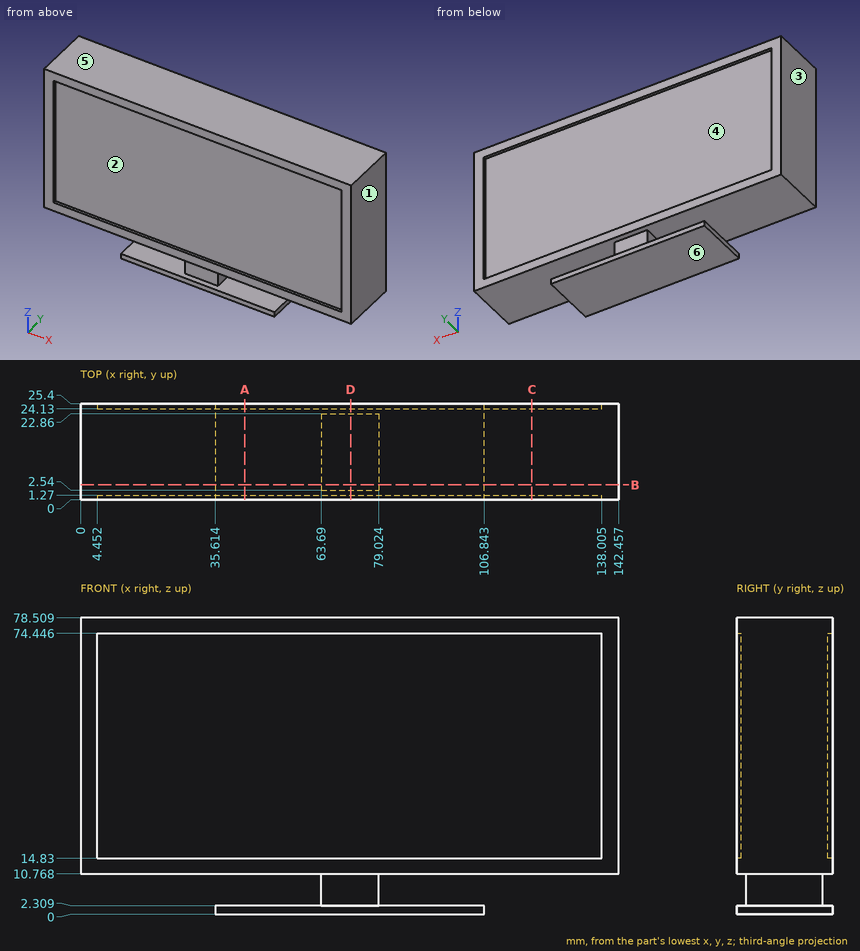
Verification items for this drawing (mm, ordinates from the low corner). A direction names the side the tool comes from. Round coordinates to 2 decimals unless told otherwise and drop trailing zeros. Order: outer loops, then holes, each group sorted by start corner. A loop starts at its lowest first (then second) coordinate and runs counter-clockwise, first axis right, second up. Notation, with made-up numbers: (23.25, 17.25) - (63.25, 17.25) arc R19 ccw to (63.25, 52.25) - close; hole circle Ø6 at (75, -34.5). An arc over 180 degrees is marked (long way). Use CSV: the item, a comma, the result in double quotes.
(1) Access from +Z, -Z, +X, -X, +Y, -Y to the whole of each face (thin tool, end or side, straight path). Record for the marked faces 1 and 2.
Entries:
face 1,"+Z, -Z, +X, +Y, -Y"
face 2,"-Y"
(2) Section check A-A on x = 43.5. Record the boundary of the cut face in (y, z) (1 decimal), and give its area (3 significant figures).
Entries:
outline,"(0, 0) - (25.4, 0) - (25.4, 2.3) - (0, 2.3) - close; (0, 10.8) - (25.4, 10.8) - (25.4, 14.8) - (24.1, 14.8) - (24.1, 74.4) - (25.4, 74.4) - (25.4, 78.5) - (0, 78.5) - (0, 74.4) - (1.3, 74.4) - (1.3, 14.8) - (0, 14.8) - close"
area,"1,630 mm^2"
(3) Gauge pin test, flat ends, axial feed: pin 1 Ø4 at (y, z) = (15.5, 6) entering from +X; pin 2 Ø4 at (x, z) = (70, 5) entering from -Y; pin 3 Ø2.5 at (y, z) = (8.5, 7.5) entering from -X. Record the tip position at first contact, or that the pin passes through.
Entries:
pin 1,"x = 79.02"
pin 2,"y = 2.54"
pin 3,"x = 63.69"
(4) Section check B-B on y = 4. Record the boundary of the cut face in (x, z) (1 decimal).
Entries:
outline,"(0, 10.8) - (63.7, 10.8) - (63.7, 2.3) - (35.6, 2.3) - (35.6, 0) - (106.8, 0) - (106.8, 2.3) - (79, 2.3) - (79, 10.8) - (142.5, 10.8) - (142.5, 78.5) - (0, 78.5) - close"
(5) Thickness scan on probe 1 along Z at (x, y) = (41, 13.5); probe 2 along Z at (x, y) = (11.5, 7.75); probe 3 along Y at (x, z) = (63.5, 30.5). Record the ranges inside material, lowest first. Write a range as from..to.
Entries:
probe 1,"0..2.31, 10.77..78.51"
probe 2,"10.77..78.51"
probe 3,"1.27..24.13"
(6) Mould release check, pull along Z, two halves, no side actions. Record for the marked faces 3, 4, 5 and 6: released by +Z, released by -Z, zero draft, split by the parting line, or undercut.
Entries:
face 3,"zero draft"
face 4,"undercut"
face 5,"released by +Z"
face 6,"released by -Z"
(7) Section check C-C on x = 119.5. Record the boundary of the cut face in (y, z) (1 decimal).
Entries:
outline,"(0, 10.8) - (25.4, 10.8) - (25.4, 14.8) - (24.1, 14.8) - (24.1, 74.4) - (25.4, 74.4) - (25.4, 78.5) - (0, 78.5) - (0, 74.4) - (1.3, 74.4) - (1.3, 14.8) - (0, 14.8) - close"
(8) Section check D-D on x = 71.5. Record the boundary of the cut face in (y, z) (1 decimal), and give its area (3 significant figures).
Entries:
outline,"(0, 0) - (25.4, 0) - (25.4, 2.3) - (22.9, 2.3) - (22.9, 10.8) - (25.4, 10.8) - (25.4, 14.8) - (24.1, 14.8) - (24.1, 74.4) - (25.4, 74.4) - (25.4, 78.5) - (0, 78.5) - (0, 74.4) - (1.3, 74.4) - (1.3, 14.8) - (0, 14.8) - (0, 10.8) - (2.5, 10.8) - (2.5, 2.3) - (0, 2.3) - close"
area,"1,800 mm^2"
